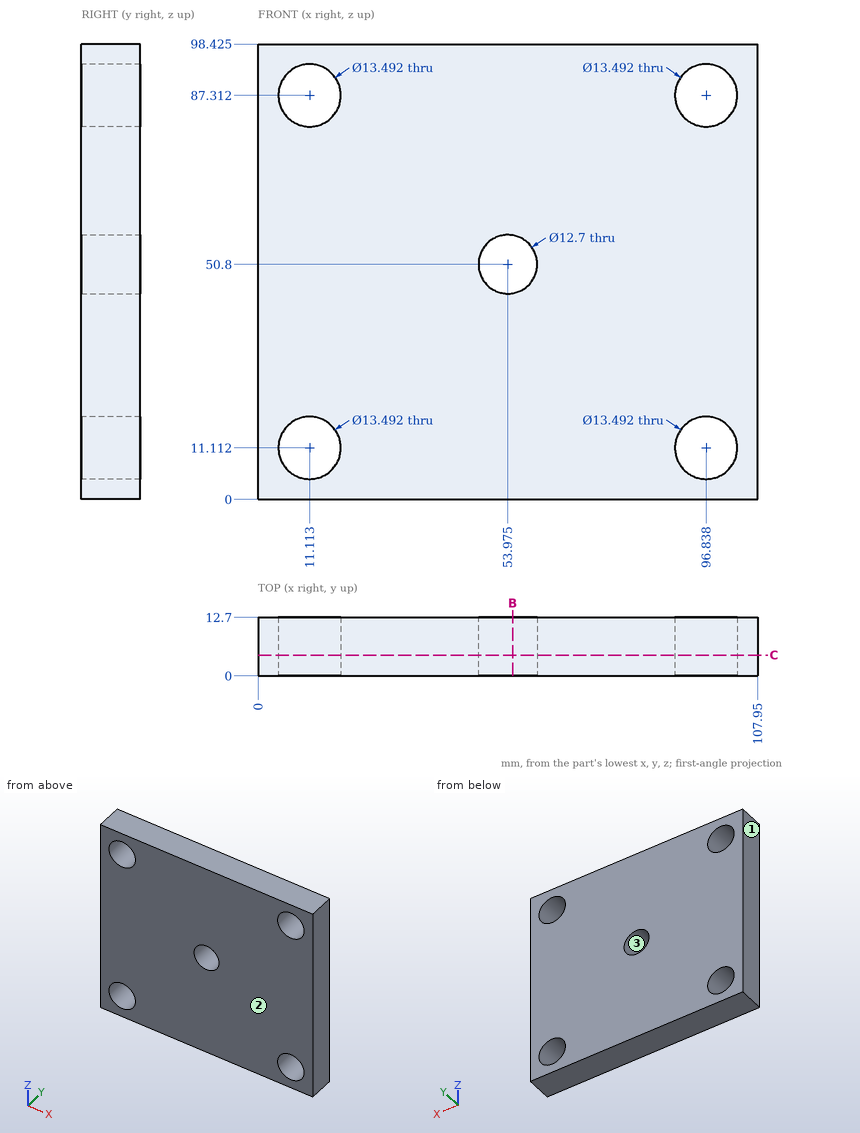
Verification items for this drawing (mm, ordinates from the low corner). Coordinates: 2 decimals unless noted, no trailing zeros. Loops run counter-clockwise (first coordinate to the right, second up) from the corner with the lowest first, then second, coordinate; pieces in that order, holes last.
Item 1: Sectioned sample at B-B, the plane x = 55. Record the boundary of the cut face in (y, z) (1 decimal), then the cut area to 3 significant figures.
Item 2: Sectioned sample at C-C, the plane y = 4.5. Count the separate pieces of the cut face and the enclosed holes in it, then the cut area to 3 significant figures.
Item 3: Release check for a two-part mould opening along X. For the marked faces 1, 2 and 3 record: released by +X, released by -X, zero draft, split by the parting line, or undercut.
Item 4: Go/stop test with a flat-tipped pin: pin 1 Ø21.5 at (x, z) = (96.84, 87.31) entering from -Y. Record where the tip stops, or that it passes through.
Item 5: Thickness scan on line 1 (Z direction, x = 94, y = 9.5) (1 decimal); line 2 (X direction, y = 12, z = 9.5); line 3 (Z direction, x = 100, y = 11.25) (1 decimal). Record the ranges inside material, lowest first.
Check result:
1. outline: (0, 0) - (12.7, 0) - (12.7, 44.5) - (0, 44.5) - close; (0, 57.1) - (12.7, 57.1) - (12.7, 98.4) - (0, 98.4) - close
1. area: 1,090 mm2
2. separate pieces: 1
2. enclosed holes: 5
2. area: 9,930 mm2
3. face 1: released by -X
3. face 2: zero draft
3. face 3: undercut
4. pin 1: stops at y = 0
5. line 1: z = 0 to 5, 17.2 to 81.2, 93.4 to 98.4
5. line 2: x = 0 to 4.56, 17.66 to 90.29, 103.39 to 107.95
5. line 3: z = 0 to 5.2, 17.1 to 81.4, 93.3 to 98.4
